from build123d import *

# Parameters (mm, degrees)
SKETCH11_W          = 12.7
SKETCH11_H          = 40
BOSS_EXTRUDE2_DEPTH = 76.2
SKETCH12_R          = 6.35
CUT_EXTRUDE5_DEPTH  = 13.7
SKETCH13_R          = 0.95
CUT_EXTRUDE6_DEPTH  = 30
SKETCH17_R          = 0.95
CUT_EXTRUDE8_DEPTH  = 21


with BuildPart() as part:
    # Sketch11 → Boss-Extrude2 (new body)
    with BuildSketch(Plane(origin=(0, 0, 0), x_dir=(1, 0, 0), z_dir=(0, 1, 0))):
        with Locations((6.35, -8.031139822)):
            Rectangle(SKETCH11_W, SKETCH11_H)
    extrude(amount=BOSS_EXTRUDE2_DEPTH)

    # Sketch12 → Cut-Extrude5 (cut, through all)
    with BuildSketch(Plane(origin=(12.7, 0, 0), x_dir=(0, 0, -1), z_dir=(1, 0, 0))):
        with Locations((-8.031139822, 54.5)):
            Circle(SKETCH12_R)
    extrude(amount=-CUT_EXTRUDE5_DEPTH, mode=Mode.SUBTRACT)

    # Sketch13 → Cut-Extrude6 (cut)
    with BuildSketch(Plane(origin=(0, 76.2, 0), x_dir=(1, 0, 0), z_dir=(0, 1, 0))):
        with Locations((6.35, -8.031139822)):
            Circle(SKETCH13_R)
    extrude(amount=-CUT_EXTRUDE6_DEPTH, mode=Mode.SUBTRACT)

    # Sketch17 → Cut-Extrude8 (cut)
    with BuildSketch(Plane.XZ):
        with Locations((6.35, 14.698139822)):
            Circle(SKETCH17_R)
        with Locations((6.35, 1.364139822)):
            Circle(SKETCH17_R)
    extrude(amount=-CUT_EXTRUDE8_DEPTH, mode=Mode.SUBTRACT)


solid = part.part
Design review of the part built by this model. Coordinates are the model's own, in mm. A direction names the side the tool comes from. Give positions to 0.01 mm unless a question says otherwise; leave off trailing zeros. Order: outer loops, then holes, each group sorted by start corner. A loop starts at its lowest first (then second) coordinate and runs counter-clockwise, first axis right, second up. Notation, with made-up numbers: (-17, 68) - (35, 68) arc R38 ccw to (35, 106) - close; hole circle Ø8 at (66, 45.25). An arc over 180 degrees is marked (long way). Write item = value, one per line. Start each with the question number.
Q1. Tool access review of faces 4 (the face through (6, 21, 1)), 5 (the face through (8, 76.2, 8)), 6 (the face through (6.86, 47.22, 7.23)): name each direction out of +Z, -Z, +X, -X, +Y, -Y from which nothing blocks a thin tool from reaching the whole face with its end or side.
Q2. We need section B-B on x = 6.35. State the section outline as (y, z) points, plus the area to 3 significant figures.
Q3. To check wall thickness, follow L1, parallel to Z at x = 6.5, y = 17.5; L2, parallel to Y at x = 9.5, z = 8; L3, parallel to Z at x = 7, y = 3. State the ranges of each line that lie inside material, in increasing order. Write a range as from..to.
Q4. We need section A-A on y = 54.5. State the section outline as (x, z) points, plus the area to 3 significant figures.
Q5. Mouldability with a two-part tool opening along Y and no side actions: class faces 1 (the face through (12.7, 38, 8)), 2 (the face through (6.4, 48.3, 9.4)), 3 (the face through (6, 0, 8)) as released by +Y, released by -Y, zero draft, split by the parting line, or undercut.
Q6. Clearance check with flat-ended pins moving along their axes: pin 1 Ø1.1 at (x, z) = (6.35, 8.03) entering from -Y; pin 2 Ø0.6 at (x, z) = (6.5, 8) entering from +Y; pin 3 Ø1 at (x, z) = (6.5, 1.5) entering from -Y. State where each tip first meets the part, or that it passes through.
Q7. We need section C-C on z = 4.5. State the section outline as (x, y) points.
Working result:
q1.face_4 = -Y
q1.face_5 = +Z, -Z, +X, -X, +Y
q1.face_6 = +Y
q2.outline = (0, -11.97) - (76.2, -11.97) - (76.2, 7.08) - (60.78, 7.08) arc R6.35 cw to (48.22, 7.08) - (46.2, 7.08) - (46.2, 8.98) - (48.22, 8.98) arc R6.35 cw to (60.78, 8.98) - (76.2, 8.98) - (76.2, 28.03) - (0, 28.03) - (0, 15.65) - (21, 15.65) - (21, 13.75) - (0, 13.75) - (0, 2.31) - (21, 2.31) - (21, 0.41) - (0, 0.41) - close
q2.area = 2,810 mm²
q3.L1 = -11.97..0.43, 2.3..13.76, 15.64..28.03
q3.L2 = 0..48.15, 60.85..76.2
q3.L3 = -11.97..0.67, 2.06..14.01, 15.39..28.03
q4.outline = (0, -11.97) - (12.7, -11.97) - (12.7, 1.68) - (0, 1.68) - close; (0, 14.38) - (12.7, 14.38) - (12.7, 28.03) - (0, 28.03) - close
q4.area = 347 mm²
q5.face_1 = zero draft
q5.face_2 = undercut
q5.face_3 = released by -Y
q6.pin_1 = 0
q6.pin_2 = 46.2
q6.pin_3 = 21
q7.outline = (0, 0) - (12.7, 0) - (12.7, 49.22) - (0, 49.22) - close; (0, 59.78) - (12.7, 59.78) - (12.7, 76.2) - (0, 76.2) - close
